Check sheet for the drawn part. Datum: minimum x, y, z corner. Units: mm. A direction names the side the tool comes from. Round coordinates to 2 decimals unless told otherwise and drop trailing zeros. Loops run counter-clockwise (first coordinate to the right, second up) from the corner with the lowest first, then second, coordinate; pieces in that order, holes last.
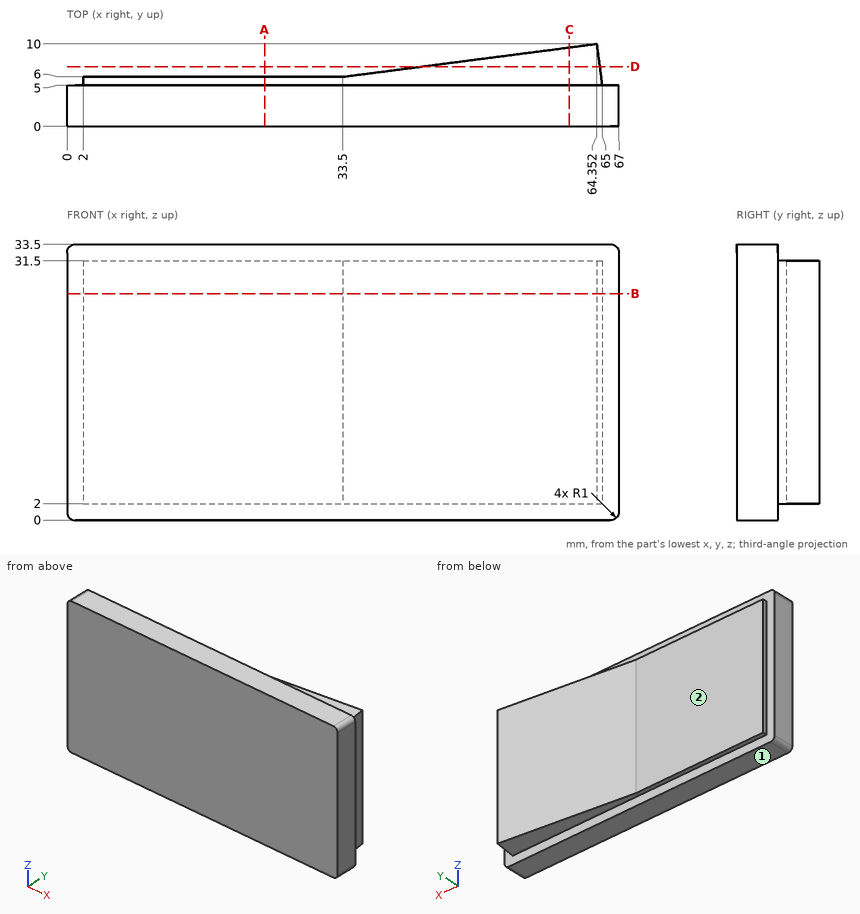
1) Sectioned sample at C-C, the plane x = 61. Record the cut outline in (y, z) (1 decimal), then the cut area to 3 significant figures.
Report:
outline: (0, 0) - (5, 0) - (5, 2) - (9.6, 2) - (9.6, 31.5) - (5, 31.5) - (5, 33.5) - (0, 33.5) - close
area: 302 mm2
2) Sectioned sample at A-A, the plane x = 24. Record the cut outline in (y, z), then the cut area to 3 significant figures.
Report:
outline: (0, 0) - (5, 0) - (5, 2) - (6, 2) - (6, 31.5) - (5, 31.5) - (5, 33.5) - (0, 33.5) - close
area: 197 mm2
3) Gauge pin test, flat ends, axial feed: pin 1 (2.5 mm diameter, centred on x = 47.5, y = 7, fed in from -Z); pin 2 (1.5 mm diameter, centred on x = 46, z = 19.5, fed in from +Y); pin 3 (5.5 mm diameter, centred on x = 42.5, y = 8.5, fed in from +Z). Record the tip position at first contact, or that the pin passes through.
Report:
pin 1: stops at z = 2
pin 2: stops at y = 7.72
pin 3: stops at z = 31.5
4) Access from +Z, -Z, +X, -X, +Y, -Y to the whole of each face (thin tool, end or side, straight path). Record for the marked faces 1 and 2.
Report:
face 1: -Z, +X, -X, +Y, -Y
face 2: +Z, -Z, -X, +Y
5) Sectioned sample at B-B, the plane z = 27.5. Record the cut outline in (x, y), then the cut area to 3 significant figures.
Report:
outline: (0, 0) - (67, 0) - (67, 5) - (65, 5) - (64.35, 10) - (33.5, 6) - (2, 6) - (2, 5) - (0, 5) - close
area: 461 mm2
6) Sectioned sample at D-D, the plane y = 7.25. Record the cut outline in (x, z), then the cut area to 3 significant figures.
Report:
outline: (43.14, 2) - (64.71, 2) - (64.71, 31.5) - (43.14, 31.5) - close
area: 636 mm2
7) Scan lines: line 1 along Y through (x, z) = (7.5, 28); line 2 along Z through (x, y) = (64, 8); line 3 along Y through (x, z) = (55, 23). Record each from-to range of solid material in increasing order.
Report:
line 1: y = 0 to 6
line 2: z = 2 to 31.5
line 3: y = 0 to 8.79
